from build123d import *

# Parameters (mm, degrees)
SKETCH1_W           = 20
SKETCH1_H           = 35
BOSS_EXTRUDE1_DEPTH = 50
SKETCH2_W           = 20
SKETCH2_H           = 55
BOSS_EXTRUDE2_DEPTH = 5
SKETCH3_W           = 27
SKETCH3_H           = 16
CUT_EXTRUDE1_DEPTH  = 16.5
CUT_EXTRUDE2_DEPTH  = 16.5
SKETCH5_R           = 2.75
CUT_EXTRUDE3_DEPTH  = 71.178344238
FILLET1_R           = 2


with BuildPart() as part:
    # Sketch1 → Boss-Extrude1 (new body)
    with BuildSketch(Plane(origin=(0, 0, 0), x_dir=(0, 0, -1), z_dir=(1, 0, 0))):
        with Locations((-10, 17.5)):
            Rectangle(SKETCH1_W, SKETCH1_H)
    extrude(amount=BOSS_EXTRUDE1_DEPTH)

    # Sketch2 → Boss-Extrude2 (add)
    with BuildSketch(Plane(origin=(50, 0, 0), x_dir=(0, 0, -1), z_dir=(1, 0, 0))):
        with Locations((-10, 17.5)):
            Rectangle(SKETCH2_W, SKETCH2_H)
    extrude(amount=BOSS_EXTRUDE2_DEPTH)

    # Sketch3 → Cut-Extrude1 (cut)
    with BuildSketch(Plane(origin=(0, 0, 0), x_dir=(-1, 0, 0), z_dir=(0, 0, -1))):
        with Locations((-20.480792353, 17.5)):
            Rectangle(SKETCH3_W, SKETCH3_H)
    extrude(amount=-CUT_EXTRUDE1_DEPTH, mode=Mode.SUBTRACT)

    # Sketch4 → Cut-Extrude2 (cut)
    with BuildSketch(Plane(origin=(0, 0, 16.5), x_dir=(-1, 0, 0), z_dir=(0, 0, -1))):
        with BuildLine():
            Line((-6.980792353, 21.5), (-6.980792353, 13.5))
            ThreePointArc((-6.980792353, 13.5), (-10.980792353, 9.5), (-14.980792353, 13.5))
            Line((-14.980792353, 13.5), (-14.980792353, 21.5))
            ThreePointArc((-14.980792353, 21.5), (-10.980792353, 25.5), (-6.980792353, 21.5))
        make_face()
    extrude(amount=-CUT_EXTRUDE2_DEPTH, mode=Mode.SUBTRACT)

    # Sketch5 → Cut-Extrude3 (cut, through all)
    with BuildSketch(Plane.ZY.offset(-50)):
        with Locations((10, 40)):
            Circle(SKETCH5_R)
        with Locations((10, -5)):
            Circle(SKETCH5_R)
    extrude(amount=-CUT_EXTRUDE3_DEPTH, mode=Mode.SUBTRACT)

    # Fillet1
    fillet1_edges = [part.edges().sort_by_distance(p)[0] for p in [
        (50, -10, 10),
        (50, -5, 0),
        (50, 40, 0),
        (52.5, -10, 0),
        (50, 45, 10),
        (52.5, 45, 0),
        (55, -10, 10),
        (55, 17.5, 0),
        (55, 45, 10),
        (33.980792353, 9.5, 8.25),
        (33.980792353, 25.5, 8.25),
        (6.980792353, 25.5, 8.25),
        (6.980792353, 9.5, 8.25),
        (33.980792353, 17.5, 0),
        (20.480792353, 9.5, 0),
        (6.980792353, 17.5, 0),
        (20.480792353, 25.5, 0),
        (0, 35, 10),
        (0, 17.5, 0),
        (0, 0, 10),
        (0, 17.5, 20),
        (25, 35, 0),
        (25, 0, 0),
    ]]
    fillet(fillet1_edges, radius=FILLET1_R)


solid = part.part
Work out the finished part from the listing and answer in its coordinate system (mm). A direction names the side the tool comes from. Coordinates: 2 decimals unless noted, no trailing zeros. Loops run counter-clockwise (first coordinate to the right, second up) from the corner with the lowest first, then second, coordinate; pieces in that order, holes last. Notation, with made-up numbers: M -35,10.5 L -4,10.5 A19 cw -4,34.5 Z; hole C -21,70.5 d11. An arc over 180 degrees is marked long. Answer in a Markdown table with one row per item. Add a question column.
1. Consider L1, parallel to Y at x = 52.75, z = 10; L2, parallel to X at y = 13.5, z = 9.75; L3, parallel to Y at x = 12.5, z = 3.25. Determine where each line is inside the solid, lowest interval first.
2. Flat-ended cylindrical pins translate along their axes: P1, Ø9, axis at y = 39, z = 9.5, coming from the -X side; P2, Ø4.5, axis at x = 9.5, y = 22.5, coming from the -Z side; P3, Ø7, axis at y = 40, z = 10, coming from the -X side; P4, Ø3, axis at x = 11, y = 22, coming from the -Z side. Find the tip coordinate at first contact, or state that the pin passes through.
3. The mould has two halves that part along X. Classify faces 1 (the flat face through (6.981, 18, 11)), 2 (the cylindrical face through (50.57, -4.04, 0.6)), 3 (the cylindrical face through (27.35, 0.57, 0.6)): pulls with the +X half, pulls with the -X half, needs draft (parallel to the pull), parting line crosses it, or undercut.
4. Find section B-B, the plane y = 16.5. Write down the section's boundary in (x, z).
5. Find section D-D, the plane x = 47.5. Write down the section's boundary in (y, z).
6. Find section A-A, the plane z = 10. State how many separate pieces and enclosed holes the cut face has, then the cut area to 3 significant figures.
7. Find section C-C, the plane x = 10. Write down the section's boundary in (y, z), then the cut area to 3 significant figures.
8. A tool of negligible diameter and unlimited length cuts with its end or side. For faces 4 (the flat face through (26, 0, 11)), 5 (the cylindrical face through (50.57, 39.18, 0.6)), 6 (the flat face through (21, 25.5, 9)), 7 (the cylindrical face through (10.9, 9.5, 18.2)), 8 (the flat face through (50, 37, 11)), from which of +Z, -Z, +X, -X, +Y, -Y can it reach the whole face along a straight path? Write none if from no direction.
Reported:
| question | item | result |
|---|---|---|
| 1 | L1 | y = -10 to -7.75, -2.25 to 37.25, 42.75 to 45 |
| 1 | L2 | x = 0 to 6.98, 33.98 to 55 |
| 1 | L3 | y = 0 to 9.5, 25.5 to 35 |
| 2 | P1 | stops at x = 0.68 |
| 2 | P2 | stops at z = 16.5 |
| 2 | P3 | stops at x = 50 |
| 2 | P4 | passes through |
| 3 | face 1 | undercut |
| 3 | face 2 | pulls with the -X half |
| 3 | face 3 | needs draft |
| 4 | outline | M 0,2 A2 ccw 2,0 L 4.98,0 A2 ccw 6.98,2 L 6.98,20 L 2,20 A2 ccw 0,18 Z; M 14.98,16.5 L 33.98,16.5 L 33.98,2 A2 ccw 35.98,0 L 53,0 A2 ccw 55,2 L 55,20 L 14.98,20 Z |
| 5 | outline | M 0,2 A2 ccw 2,0 L 33,0 A2 ccw 35,2 L 35,20 L 0,20 Z |
| 6 | separate pieces | 3 |
| 6 | enclosed holes | 1 |
| 6 | area | 1,540 mm^2 |
| 7 | outline | M 0,2 A2 ccw 2,0 L 7.5,0 A2 ccw 9.5,2 L 9.5,16.5 L 9.62,16.5 L 9.62,20 L 0,20 Z; M 25.38,16.5 L 25.5,16.5 L 25.5,2 A2 ccw 27.5,0 L 33,0 A2 ccw 35,2 L 35,20 L 25.38,20 Z |
| 7 | area | 377 mm^2 |
| 8 | face 4 | +Z, -Z, -X, -Y |
| 8 | face 5 | -Z, -X, +Y |
| 8 | face 6 | -Z |
| 8 | face 7 | +Z, -Z |
| 8 | face 8 | +Z, -Z, -X, +Y |
